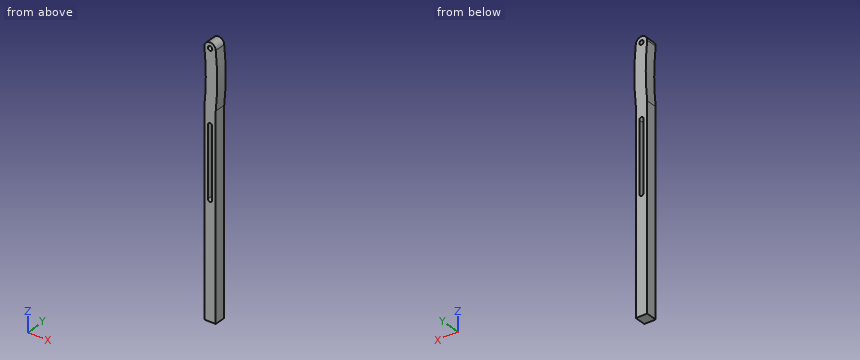
Autodesk Inventor part; units mm, degrees
ref_plane "XZ Plane" through (0, 0, 0) normal (0, 1, 0) x (-1, 0, 0)
ref_plane "XY Plane" through (0, 0, 0) normal (0, 0, 1) x (1, 0, 0)
sketch "Sketch1" plane through (0, 0, 0) normal (0, 1, 0) x (-1, 0, 0)
  line L0 (0, 0) -> (0, -319.927) construction
  line L1 (-4, 0) -> (-4, -319.927)
  line L2 (4, -319.927) -> (4, 0)
  arc A0 (4, 0) -> (-4, 0) centre (0, 0) ccw
  arc A1 (-4, -319.927) -> (4, -319.927) centre (0, -319.927) ccw
  circle A2 centre (0, 0) radius 1.5
  circle A3 centre (0, -319.927) radius 1.5
  line L3 (0, -50.8) -> (0, -100) construction
  line L4 (-1.5, -50.8) -> (-1.5, -100)
  line L5 (1.5, -100) -> (1.5, -50.8)
  arc A4 (1.5, -50.8) -> (-1.5, -50.8) centre (0, -50.8) ccw
  arc A5 (-1.5, -100) -> (1.5, -100) centre (0, -100) ccw
  arc A6 (4, 0) -> (4, -40) centre (202.9975, -20) ccw
  arc A7 (-4, 0) -> (-4, -40) centre (194.9975, -20) ccw
  point P0 (0, -159.9635)
  point P1 (0, -75.4)
  dimension "d0" = 319.927
  dimension "d1" = 8
  dimension "d2" = 3
  dimension "d3" = 3
  dimension "d12" = 3
  dimension "d13" = 50.8
  dimension "d14" = 100
  dimension "d15" = 40
  dimension "d16" = 200
  dimension "d17" = 200
extrude "Extrusion1" add sketch "Sketch1" along normal blind 8 contours A0 A6 L2 A1 L1 | L1 A7
sketch "Sketch2" plane through (0, 0, 0) normal (0, -1, 0) x (1, 0, 0)
  arc A0 (4, -40) -> (4, 0) centre (-194.9975, -20) ccw
  arc A1 (4, 0) -> (-4, 0) centre (0, 0) ccw
  arc A2 (-4, -40) -> (-4, 0) centre (-202.9975, -20) ccw
  line L0 (-4, -319.927) -> (-4, -40)
  arc A3 (-4, -319.927) -> (4, -319.927) centre (0, -319.927) ccw
  line L1 (4, -40) -> (4, -319.927)
  circle A4 centre (0, 0) radius 1.5
  circle A5 centre (0, -319.927) radius 1.5
  arc A6 (1.5, -50.8) -> (-1.5, -50.8) centre (0, -50.8) ccw
  line L2 (1.5, -100) -> (1.5, -50.8)
  arc A7 (-1.5, -100) -> (1.5, -100) centre (0, -100) ccw
  line L3 (-1.5, -50.8) -> (-1.5, -100)
sketch "Sketch3" plane through (0, 8, 0) normal (0, 1, 0) x (1, 0, 0)
  line L0 (-21.634, 180.7321) -> (39.8396, 180.7321)
  line L1 (39.8396, 180.7321) -> (39.8396, -20.7362)
  line L2 (39.8396, -20.7362) -> (-21.634, -20.7362)
  line L3 (-21.634, -20.7362) -> (-21.634, 180.7321)
  line L4 (-50.5628, 342.9399) -> (62.0528, 342.9399)
  line L5 (62.0528, 342.9399) -> (62.0528, -55.3474)
  line L6 (62.0528, -55.3474) -> (-50.5628, -55.3474)
  line L7 (-50.5628, -55.3474) -> (-50.5628, 342.9399)
  point P0 (0, 0)
extrude "Extrusion2" cut sketch "Sketch3" along normal mid plane 20
sketch "Sketch4" plane through (0, 8, 0) normal (0, 1, 0) x (1, 0, 0)
  line L0 (4, 180.7321) -> (-4, 180.7321)
  line L1 (-4, 180.7321) -> (-4, 40)
  arc A0 (-4, 0) -> (-4, 40) centre (-202.9975, 20) ccw
  arc A1 (-4, 0) -> (4, 0) centre (0, 0) ccw
  arc A2 (4, 0) -> (4, 40) centre (-194.9975, 20) ccw
  line L2 (4, 40) -> (4, 180.7321)
  circle A3 centre (0, 0) radius 1.5
  arc A4 (-1.5, 50.8) -> (1.5, 50.8) centre (0, 50.8) ccw
  line L3 (-1.5, 50.8) -> (-1.5, 100)
  arc A5 (1.5, 100) -> (-1.5, 100) centre (0, 100) ccw
  line L4 (1.5, 100) -> (1.5, 50.8)
properties part number "Part_8_p1"
The model under review builds one solid part; all positions refer to its coordinate system, in mm. Round coordinates to 2 decimals unless told otherwise and drop trailing zeros. Write each loop counter-clockwise with the first axis right and the second up, starting at its lowest first coordinate (ties: lowest second). Pieces come first, ordered by that corner, then holes.
(1) We need section B-B on y = 2.25. Give the boundary of the cut face in (x, z).
(2) Wall thickness on L1, parallel to Z at x = 0, y = 6; L2, parallel to X at y = 7.5, z = -65.5; L3, parallel to Z at x = 1, y = 4.75: over which ranges is each line inside the solid? List them lowest first.
(3) We need section A-A on x = 0. Give the boundary of the cut face in (y, z).
(4) Insertion check: pin 1 (2.5 mm diameter, centred on y = 5, z = -110.5, fed in from +X); pin 2 (3 mm diameter, centred on x = 3, y = 6.5, fed in from +Z); pin 3 (3 mm diameter, centred on x = 2, y = 5.5, fed in from +Z). Each pin has a flat end and moves straight along its axis. Give the tip position at first contact, or say it passes through.
(5) We need section C-C on z = -108.5. Give the boundary of the cut face in (x, y).
Findings below:
1. outline: (-4, -180.73) - (4, -180.73) - (4, -40) arc R200 ccw to (4, 0) arc R4 ccw to (-4, 0) arc R200 cw to (-4, -40) - close; hole (-1.5, -100) arc R1.5 ccw to (1.5, -100) - (1.5, -50.8) arc R1.5 ccw to (-1.5, -50.8) - close; hole circle Ø3 at (0, 0)
2. L1: z = -180.73 to -101.5, -49.3 to -1.5, 1.5 to 4
2. L2: x = -4 to -1.5, 1.5 to 4
2. L3: z = -180.73 to -101.12, -49.68 to -1.12, 1.12 to 3.87
3. outline: (0, -180.73) - (8, -180.73) - (8, -101.5) - (0, -101.5) - close; (0, -49.3) - (8, -49.3) - (8, -1.5) - (0, -1.5) - close; (0, 1.5) - (8, 1.5) - (8, 4) - (0, 4) - close
4. pin 1: stops at x = 4
4. pin 2: stops at z = 3.71
4. pin 3: stops at z = 3.97
5. outline: (-4, 0) - (4, 0) - (4, 8) - (-4, 8) - close
